Input: part model. Units: mm. Frame: model coordinates. Coordinates: 2 decimals unless noted, no trailing zeros. Write each loop counter-clockwise with the first axis right and the second up, starting at its lowest first coordinate (ties: lowest second). Pieces come first, ordered by that corner, then holes. Notation, with made-up numbers: (25, 82.25) - (68, 82.25) arc R36 cw to (68, 120.25) - close; hole circle Ø8 at (79.25, -35). An arc over 180 degrees is marked (long way). Use a Markdown table: item, result. Add a question column.
Q1. Section query C-C (z = -29). Return the cut outline in (x, y).
Q2. Pin query (flat end, axial travel): P1, Ø3.5, axis at x = -85, z = -10, coming from the -Y side; P2, Ø6, axis at y = 4.5, z = -27, coming from the +X side. Return the tip coordinate at first contact, or that it passes through.
Q3. Mould query, pull axis Z, two halves, no side actions, for faces 1 (the face through (-17.05, 15.21, -39.73)), 2 (the face through (-98.859, 14.79, -48.797)), 3 (the face through (-98.797, 14.79, -1.141)). Classes: released by +Z, released by -Z, zero draft, split by the parting line, or undercut.
Q4. Material intervals for probe 1 along Z at (x, y) = (-85, 12); probe 2 along X at (y, z) = (24, -10); probe 3 along X at (y, z) = (2, -41), sorted ascending. Write a range as from..to.
Q5. Section query A-A (x = -85). Return the cut outline in (y, z).
Q6. Section query D-D (x = -50). Return the cut outline in (y, z), then the cut area to 3 significant figures.
Q7. Section query B-B (z = -10). Return the cut outline in (x, y), then the cut area to 3 significant figures.
Autodesk Inventor part; units mm, degrees
ref_plane "YZ Plane" through (0, 0, 0) normal (1, 0, 0) x (0, 1, 0)
ref_plane "XZ Plane" through (0, 0, 0) normal (0, 1, 0) x (-1, 0, 0)
ref_plane "XY Plane" through (0, 0, 0) normal (0, 0, 1) x (1, 0, 0)
sketch "Skizze2" plane through (0, 0, 0) normal (0, 1, 0) x (-1, 0, 0)
  line L0 (0, -4) -> (0, -46)
  line L1 (4, -50) -> (96, -50)
  line L2 (100, -46) -> (100, -4)
  line L3 (96, 0) -> (4, 0)
  arc A0 (100, -4) -> (96, 0) centre (96, -4) ccw
  arc A1 (96, -50) -> (100, -46) centre (96, -46) ccw
  arc A2 (0, -46) -> (4, -50) centre (4, -46) ccw
  arc A3 (4, 0) -> (0, -4) centre (4, -4) ccw
  point P0 (0, 0)
  point P1 (0, -50)
  point P2 (100, -50)
  point P3 (100, 0)
  dimension "breite" = 50
  dimension "länge" = 100
  dimension "d11" = 50
  dimension "radius" = 4
extrude "Extrusion2" add sketch "Skizze2" along normal blind 30
sketch "Skizze4" plane through (-96, 0, 0) normal (0, 0, 1) x (1, 0, 0)
  point P0 (96, 0)
sketch "Skizze5" plane through (-96, 0, 0) normal (0, 0, 1) x (1, 0, 0)
  line L0 (0, 0) -> (0, 30)
  line L1 (0, 0) -> (46, 0)
  line L2 (92, 0) -> (0, 0)
  circle A0 centre (46, 0) radius 10
  point P0 (96, 0)
  dimension "d15" = 20
extrude "Extrusion3" cut sketch "Skizze5" against normal through all
sketch "Skizze6" plane through (0, 0, 0) normal (0, -1, 0) x (1, 0, 0)
  line L0 (0, 0) -> (0, -10)
  line L1 (0, -4) -> (0, -46)
  line L2 (0, -10) -> (-15, -10)
  line L3 (-15, -10) -> (-85, -10)
  line L4 (-85, -10) -> (-85, -40)
  line L5 (-85, -40) -> (-15, -40)
  dimension "d18" = 10
  dimension "d19" = 15
  dimension "d20" = 70
  dimension "d21" = 30
  dimension "d22" = 70
hole "Bohrung1" at (-15, 0, -40) at (-15, 0, -10) at (-85, 0, -40) at (-85, 0, -10) direction (0, 1, 0) diameter 4.134 end through all
equation "\"d15\" = durchmesser"
properties part number "TrittUT" material "PVC, hart"
Values follow:
| question | item | result |
|---|---|---|
| 1 | outline | (-100, 0) - (-60, 0) arc R10 cw to (-40, 0) - (0, 0) - (0, 30) - (-100, 30) - close |
| 2 | P1 | through |
| 2 | P2 | x = 0 |
| 3 | face 1 | undercut |
| 3 | face 2 | released by -Z |
| 3 | face 3 | released by +Z |
| 4 | probe 1 | -50..-42.07, -37.93..-12.07, -7.93..0 |
| 4 | probe 2 | -100..-87.07, -82.93..-17.07, -12.93..0 |
| 4 | probe 3 | -100..-86.81, -83.19..-59.8, -40.2..-16.81, -13.19..0 |
| 5 | outline | (0, -50) - (30, -50) - (30, -42.07) - (0, -42.07) - close; (0, -37.93) - (30, -37.93) - (30, -12.07) - (0, -12.07) - close; (0, -7.93) - (30, -7.93) - (30, 0) - (0, 0) - close |
| 6 | outline | (10, -50) - (30, -50) - (30, 0) - (10, 0) - close |
| 6 | area | 1,000 mm2 |
| 7 | outline | (-100, 0) - (-87.07, 0) - (-87.07, 30) - (-100, 30) - close; (-82.93, 0) - (-60, 0) arc R10 cw to (-40, 0) - (-17.07, 0) - (-17.07, 30) - (-82.93, 30) - close; (-12.93, 0) - (0, 0) - (0, 30) - (-12.93, 30) - close |
| 7 | area | 2,590 mm2 |
